```python
from build123d import *

# Parameters (mm, degrees)
F1_DEPTH = 100
F3_DEPTH = 3
F5_DEPTH = 8
F6_W     = 30
F6_H     = 35
F7_DEPTH = 2
F8_W     = 30
F8_H     = 35
F9_DEPTH = 2


with BuildPart() as f1:
    # F0 (on Top) → F1 (new body)
    with BuildSketch(Plane.XY):
        Polygon((-165, -100), (0, -100), (0, -70), (-20, -70), (-20, -30), (0, -30), (0, 30), (20, 30), (20, 70), (0, 70), (0, 100), (-165, 100), align=None)
        Polygon((-2.999997, -97.000003), (-162.000003, -97.000003), (-162.000003, 97.000003), (-2.999997, 97.000003), (-2.999997, 67.000003), (17.000003, 67.000003), (17.000003, 32.999997), (-2.999997, 32.999997), (-2.999997, -27.000003), (-22.999997, -27.000003), (-22.999997, -72.999997), (-2.999997, -72.999997), align=None, mode=Mode.SUBTRACT)
    extrude(amount=F1_DEPTH)

    # F2 (on face) → F3 (join)
    with BuildSketch(Plane.XY.offset(100)):
        Polygon((-165, 100), (-165, -100), (0, -100), (0, -70), (-20, -70), (-20, -30), (0, -30), (0, 30), (20, 30), (20, 70), (0, 70), (0, 100), align=None)
    extrude(amount=-F3_DEPTH)

    # F4 (on face) → F5 (join)
    with BuildSketch(Plane.XY.offset(100)):
        Polygon((-152, -100), (0, -100), (0, -87), (-152, -87), (-152, 100), (-165, 100), (-165, -100), (-162, -100), align=None)
    extrude(amount=F5_DEPTH)

    # F6 (on face) → F7 (cut)
    with BuildSketch(Plane.XZ.offset(100)):
        with Locations((-25, 47.5)):
            Rectangle(F6_W, F6_H)
        with Locations((-75, 47.5)):
            Rectangle(F6_W, F6_H)
        Polygon((-110, 30), (-110, 65), (-140, 65), (-140, 30), (-140, 0), (-110, 0), align=None)
    extrude(amount=-F7_DEPTH, mode=Mode.SUBTRACT)

    # F8 (on face) → F9 (cut)
    with BuildSketch(Plane(origin=(-165, 0, 0), x_dir=(0, -1, 0), z_dir=(-1, 0, 0))):
        Polygon((-15, 65), (-15, 30), (0, 30), (15, 30), (15, 65), align=None)
        with Locations((50, 47.5)):
            Rectangle(F8_W, F8_H)
        with Locations((-50, 47.5)):
            Rectangle(F8_W, F8_H)
    extrude(amount=-F9_DEPTH, mode=Mode.SUBTRACT)


solid = f1.part
```
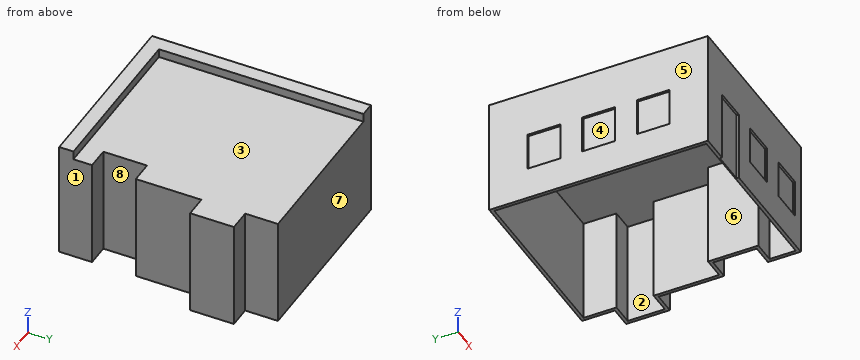
For this review, take the finished solid that the model builds, in its own axes (mm). Face numbers are marked on the shaded views. A direction names the side the tool comes from. Round coordinates to 2 decimals unless told otherwise and drop trailing zeros. Write each loop counter-clockwise with the first axis right and the second up, starting at its lowest first coordinate (ties: lowest second). Pieces come first, ordered by that corner, then holes. Notation, with made-up numbers: (45, 78) -> (84, 78) arc R29 cw to (84, 114) -> close; hole circle Ø3 at (11.5, -6.75). An arc over 180 degrees is marked (long way). One line per question, with ' | ' between items. Start each with the question number.
1) For pin 1 Ø10 at (x, y) = (-101.5, 29.5) entering from -Z; pin 2 Ø8 at (x, y) = (-27.5, -11.5) entering from +Z; pin 3 Ø2 at (y, z) = (-99, 20) entering from +X, all flat-tipped, find the tip position at first contact; note any pin that passes through.
2) Add section B-B (x = -75). Write out the cut boundary in (y, z).
3) Machinability: for the marked faces 1, 2, 3 and 4, which of the approach directions +Z, -Z, +X, -X, +Y, -Y give a long, thin tool a straight path to every point of the face, cutting with its end or side? Answer none if there is none.
4) Add section C-C (y = -12). Write out the cut boundary in (x, z), and give its area (3 significant figures).
5) Add section A-A (z = 81). Write out the cut boundary in (x, y), and give its area (3 significant figures).
6) Wall thickness on line 1 along Y through (x, z) = (-11, 45); line 2 along Y through (x, z) = (-3.5, 60); line 3 along X through (y, z) = (-84, 60.5): over which ranges is each line inside the solid? List them lowest first.
7) Mouldability with a two-part tool opening along X and no side actions: class the marked faces 5, 6, 7 and 8 as +X half, -X half, draft (parallel to the pull), parting line (faces both ways), or undercut.
8) Add section D-D (z = 8.5). Write out the cut boundary in (x, y), and give its area (3 significant figures).
Reported:
1) pin 1: stops at z = 97 | pin 2: stops at z = 100 | pin 3: stops at x = 0
2) outline: (-100, 0) -> (-97, 0) -> (-97, 97) -> (97, 97) -> (97, 0) -> (100, 0) -> (100, 100) -> (-87, 100) -> (-87, 108) -> (-100, 108) -> (-100, 65) -> (-98, 65) -> (-98, 30) -> (-100, 30) -> close
3) face 1: +Z, -Z, +X, -Y | face 2: -Z | face 3: +Z, +X, +Y | face 4: -X
4) outline: (-165, 0) -> (-162, 0) -> (-162, 97) -> (-3, 97) -> (-3, 0) -> (0, 0) -> (0, 100) -> (-152, 100) -> (-152, 108) -> (-165, 108) -> (-165, 65) -> (-163, 65) -> (-163, 30) -> (-165, 30) -> close | area: 1,110 mm²
5) outline: (-165, -100) -> (0, -100) -> (0, -70) -> (-20, -70) -> (-20, -30) -> (0, -30) -> (0, 30) -> (20, 30) -> (20, 70) -> (0, 70) -> (0, 100) -> (-165, 100) -> close; hole (-162, -97) -> (-3, -97) -> (-3, -73) -> (-23, -73) -> (-23, -27) -> (-3, -27) -> (-3, 33) -> (17, 33) -> (17, 67) -> (-3, 67) -> (-3, 97) -> (-162, 97) -> close | area: 2,390 mm²
6) line 1: y = -98 to -97, -73 to -70, -30 to -27, 97 to 100 | line 2: y = -100 to -97, -73 to -70, -30 to -27, 97 to 100 | line 3: x = -165 to -162, -3 to 0
7) face 5: -X half | face 6: undercut | face 7: draft | face 8: +X half
8) outline: (-165, -100) -> (-140, -100) -> (-140, -98) -> (-110, -98) -> (-110, -100) -> (0, -100) -> (0, -70) -> (-20, -70) -> (-20, -30) -> (0, -30) -> (0, 30) -> (20, 30) -> (20, 70) -> (0, 70) -> (0, 100) -> (-165, 100) -> close; hole (-162, -97) -> (-3, -97) -> (-3, -73) -> (-23, -73) -> (-23, -27) -> (-3, -27) -> (-3, 33) -> (17, 33) -> (17, 67) -> (-3, 67) -> (-3, 97) -> (-162, 97) -> close | area: 2,330 mm²
